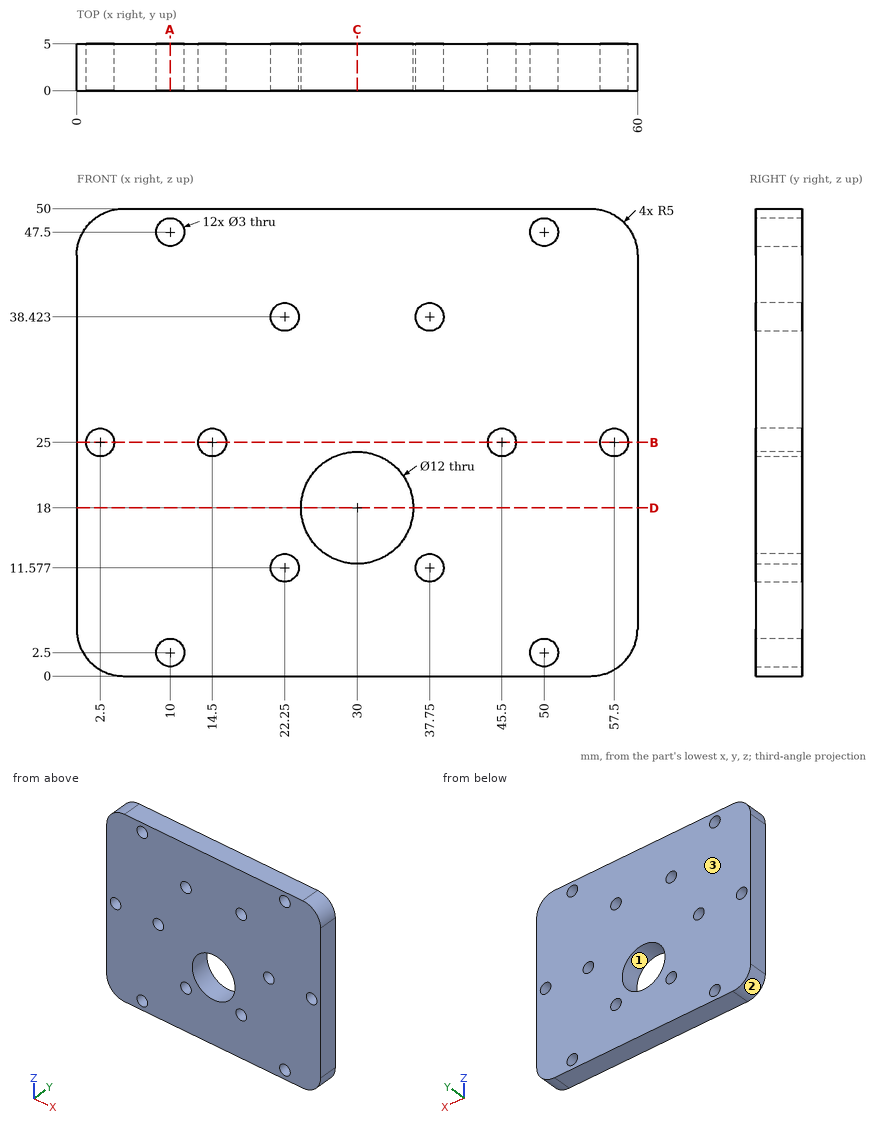
Geometry check sheet. Reference: drawing and pictorial views, mm from the part's lowest x, y, z. Give positions to 0.01 mm unless a question says otherwise; leave off trailing zeros. Loops run counter-clockwise (first coordinate to the right, second up) from the corner with the lowest first, then second, coordinate; pieces in that order, holes last. Notation, with made-up numbers: M 63,-4.5 L 96,-4.5 A24 cw 96,31.5 Z; hole C 38.5,28 d9. An arc over 180 degrees is marked long. Use a Markdown table: item, result. Add a question column.
Q1. Sectioned sample at D-D, the plane z = 18. Record the cut outline in (x, y).
Q2. Sectioned sample at B-B, the plane z = 25. Record the cut outline in (x, y), then the cut area to 3 significant figures.
Q3. Sectioned sample at C-C, the plane x = 30. Record the cut outline in (y, z).
Q4. Scan lines: line 1 along X through (y, z) = (3.9, 25); line 2 along X through (y, z) = (0.4, 47) (1 decimal); line 3 along Z through (x, y) = (51, 0.7). Record each from-to range of solid material in increasing order. Write a range as [from, to].
Q5. Mould release check, pull along X, two halves, no side actions. Record for the marked faces 1, 2 and 3: pulls with the +X half, pulls with the -X half, needs draft (parallel to the pull), parting line crosses it, or undercut.
Q6. Sectioned sample at A-A, the plane x = 10. Record the cut outline in (y, z), then the cut area to 3 significant figures.
Verdict:
| question | item | result |
|---|---|---|
| 1 | outline | M 0,0 L 24,0 L 24,5 L 0,5 Z; M 36,0 L 60,0 L 60,5 L 36,5 Z |
| 2 | outline | M 0,0 L 1,0 L 1,5 L 0,5 Z; M 4,0 L 13,0 L 13,5 L 4,5 Z; M 16,0 L 44,0 L 44,5 L 16,5 Z; M 47,0 L 56,0 L 56,5 L 47,5 Z; M 59,0 L 60,0 L 60,5 L 59,5 Z |
| 2 | area | 240 mm^2 |
| 3 | outline | M 0,0 L 5,0 L 5,12 L 0,12 Z; M 0,24 L 5,24 L 5,50 L 0,50 Z |
| 4 | line 1 | [0, 1], [4, 13], [16, 44], [47, 56], [59, 60] |
| 4 | line 2 | [0.4, 8.6], [11.4, 48.6], [51.4, 59.6] |
| 4 | line 3 | [0, 1.38], [3.62, 46.38], [48.62, 50] |
| 5 | face 1 | undercut |
| 5 | face 2 | pulls with the -X half |
| 5 | face 3 | needs draft |
| 6 | outline | M 0,0 L 5,0 L 5,1 L 0,1 Z; M 0,4 L 5,4 L 5,46 L 0,46 Z; M 0,49 L 5,49 L 5,50 L 0,50 Z |
| 6 | area | 220 mm^2 |
